Part model, mm, in its own coordinate system. Face numbers are marked on the shaded views. A direction names the side the tool comes from. Round coordinates to 2 decimals unless told otherwise and drop trailing zeros. Write each loop counter-clockwise with the first axis right and the second up, starting at its lowest first coordinate (ties: lowest second). Pieces come first, ordered by that corner, then holes.
1) Which spindle directions (+Z, -Z, +X, -X, +Y, -Y) get a long thin tool onto all of the face, cutting with end or side? Do the marked faces 1 and 2. Say none if no direction does.
2) Saw through at C-C on y = 14.25. Write the cut outline in (x, z).
3) Saw through at A-A on z = 9. Write the cut outline in (x, y).
4) Saw through at D-D on y = 4.25. Write the cut outline in (x, z).
5) Flat gauge pins, fed straight in: pin 1 (8 mm diameter, centred on x = 10, z = 94, fed in from +Y); pin 2 (6.5 mm diameter, centred on y = 12, z = 71.5, fed in from -X). Where does each tip first touch, or does it go through?
6) Drill centre lines: L1, parallel to Z at x = 10, y = 0.9; L2, parallel to Y at x = 4.5, z = 110; L3, parallel to X at y = 9.75, z = 43.5. Where is each one in solid material? Low to high.
7) Saw through at B-B on x = 10. Write the cut outline in (y, z).
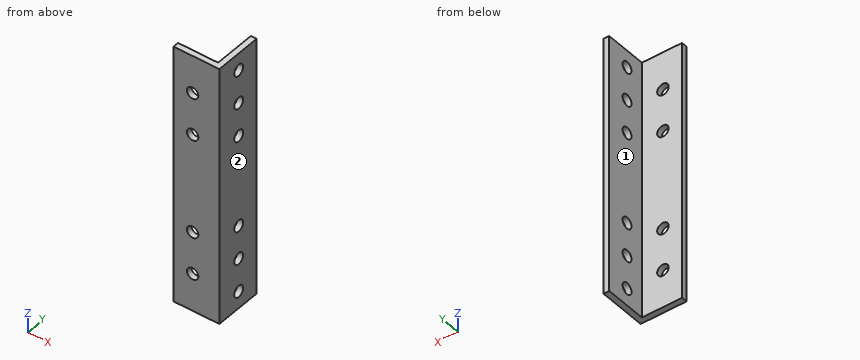
```python
from build123d import *

# Parameters (mm, degrees)
SALIENTE_EXTRUIR1_DEPTH = 136
CROQUIS2_R              = 3
CORTAR_EXTRUIR1_DEPTH   = 25
CROQUIS3_R              = 3
CORTAR_EXTRUIR2_DEPTH   = 26


with BuildPart() as part:
    # Croquis1 → Saliente-Extruir1 (new body)
    with BuildSketch(Plane.XY):
        Polygon((0, 0), (24, 0), (24, 25), (21, 25), (21, 3), (0, 3), align=None)
    extrude(amount=SALIENTE_EXTRUIR1_DEPTH)

    # Croquis2 → Cortar-Extruir1 (cut, through all)
    with BuildSketch(Plane(origin=(24, 0, 0), x_dir=(0, 0, -1), z_dir=(1, 0, 0))):
        with Locations((-127, 13)):
            Circle(CROQUIS2_R)
        with Locations((-109.5, 13)):
            Circle(CROQUIS2_R)
        with Locations((-92, 13)):
            Circle(CROQUIS2_R)
        with Locations((-9, 13)):
            Circle(CROQUIS2_R)
        with Locations((-26.5, 13)):
            Circle(CROQUIS2_R)
        with Locations((-44, 13)):
            Circle(CROQUIS2_R)
    extrude(amount=-CORTAR_EXTRUIR1_DEPTH, mode=Mode.SUBTRACT)

    # Croquis3 → Cortar-Extruir2 (cut, through all)
    with BuildSketch(Plane.XZ):
        with Locations((10, 19.8)):
            Circle(CROQUIS3_R)
        with Locations((10, 42)):
            Circle(CROQUIS3_R)
        with Locations((10, 116.2)):
            Circle(CROQUIS3_R)
        with Locations((10, 94)):
            Circle(CROQUIS3_R)
    extrude(amount=-CORTAR_EXTRUIR2_DEPTH, mode=Mode.SUBTRACT)


solid = part.part
```
Completed:
1. face 1: +Z, -Z, -X, +Y
1. face 2: +Z, -Z, +X, +Y, -Y
2. outline: (21, 0) - (24, 0) - (24, 6.27) - (21, 6.27) - close; (21, 11.73) - (24, 11.73) - (24, 23.77) - (21, 23.77) - close; (21, 29.23) - (24, 29.23) - (24, 41.27) - (21, 41.27) - close; (21, 46.73) - (24, 46.73) - (24, 89.27) - (21, 89.27) - close; (21, 94.73) - (24, 94.73) - (24, 106.77) - (21, 106.77) - close; (21, 112.23) - (24, 112.23) - (24, 124.27) - (21, 124.27) - close; (21, 129.73) - (24, 129.73) - (24, 136) - (21, 136) - close
3. outline: (0, 0) - (24, 0) - (24, 10) - (21, 10) - (21, 3) - (0, 3) - close; (21, 16) - (24, 16) - (24, 25) - (21, 25) - close
4. outline: (21, 0) - (24, 0) - (24, 136) - (21, 136) - close
5. pin 1: stops at y = 3
5. pin 2: stops at x = 21
6. L1: z = 0 to 16.8, 22.8 to 39, 45 to 91, 97 to 113.2, 119.2 to 136
6. L2: y = 0 to 3
6. L3: x = 21 to 24
7. outline: (0, 0) - (3, 0) - (3, 16.8) - (0, 16.8) - close; (0, 22.8) - (3, 22.8) - (3, 39) - (0, 39) - close; (0, 45) - (3, 45) - (3, 91) - (0, 91) - close; (0, 97) - (3, 97) - (3, 113.2) - (0, 113.2) - close; (0, 119.2) - (3, 119.2) - (3, 136) - (0, 136) - close
